Design review of the part built by this model. Coordinates are the model's own, in mm. Face numbers are marked on the shaded views. A direction names the side the tool comes from. Give positions to 0.01 mm unless a question says otherwise; leave off trailing zeros. Write each loop counter-clockwise with the first axis right and the second up, starting at its lowest first coordinate (ties: lowest second). Pieces come first, ordered by that corner, then holes. Notation, with made-up numbers: M 64,67 L 87,67 A12 cw 87,81 Z; hole C -39,56 d11. An arc over 180 degrees is marked long. One line per item, written item: value. Start each with the question number.
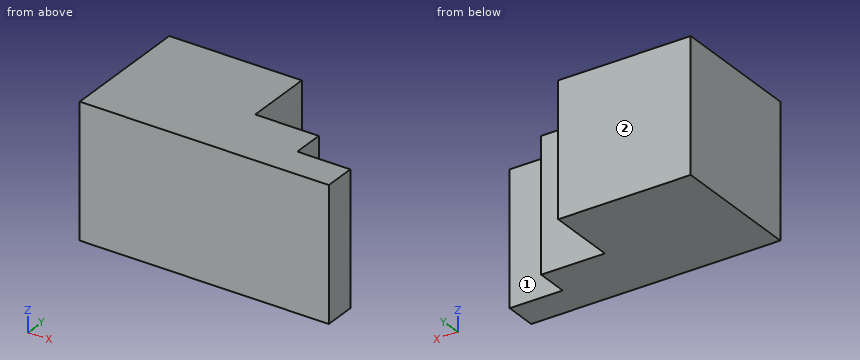
```python
from build123d import *

# Parameters (mm, degrees)
F0_W     = 10
F0_H     = 6
F1_DEPTH = 25


with BuildPart() as f1:
    # F0 (on Top) → F1 (new body)
    with BuildSketch(Plane.XY):
        Polygon((-7.03125, 25), (-32.03125, 25), (-32.03125, 0), (-7.03125, 0), (-7.03125, 12), align=None)
        Polygon((4.96875, 12), (-7.03125, 12), (-7.03125, 0), (4.96875, 0), (4.96875, 6), align=None)
        with Locations((9.96875, 3)):
            Rectangle(F0_W, F0_H)
    extrude(amount=F1_DEPTH)


solid = f1.part
```
Q1. Machinability: for the marked faces 1 and 2, which of the approach directions +Z, -Z, +X, -X, +Y, -Y give a long, thin tool a straight path to every point of the face, cutting with its end or side? Answer none if there is none.
Q2. Take a section at A-A, the plane z = 19. Give the boundary of the cut face in (x, y), then the cut area to 3 significant figures.
Q3. Take a section at B-B, the plane y = 16. Give the boundary of the cut face in (x, z), then the cut area to 3 significant figures.
Q4. For P1, Ø1.8, axis at y = 9.5, z = 13, coming from the +X side; P2, Ø6.5, axis at y = 18.5, z = 12, coming from the +X side; P3, Ø6, axis at x = -0.5, z = 18, coming from the +Y side, all flat-tipped, find the tip position at first contact; note any pin that passes through.
Q5. Wall thickness on line 1 (X direction, y = 22.75, z = 19.75); line 2 (X direction, y = 6.75, z = 6.75); line 3 (Y direction, x = 11.5, z = 14): over which ranges is each line inside the solid? List them lowest first. Write a range as from..to.
Q6. Take a section at C-C, the plane x = 3. Give the boundary of the cut face in (y, z), then the cut area to 3 significant figures.
Results list:
1. face 1: +Z, -Z, +X, +Y
1. face 2: +Z, -Z, +X, -X, +Y
2. outline: M -32.03,0 L 14.97,0 L 14.97,6 L 4.97,6 L 4.97,12 L -7.03,12 L -7.03,25 L -32.03,25 Z
2. area: 829 mm^2
3. outline: M -32.03,0 L -7.03,0 L -7.03,25 L -32.03,25 Z
3. area: 625 mm^2
4. P1: stops at x = 4.97
4. P2: stops at x = -7.03
4. P3: stops at y = 12
5. line 1: x = -32.03..-7.03
5. line 2: x = -32.03..4.97
5. line 3: y = 0..6
6. outline: M 0,0 L 12,0 L 12,25 L 0,25 Z
6. area: 300 mm^2
